from build123d import *

# Parameters (mm, degrees)
SKETCH4_R          = 1
CUT_EXTRUDE1_DEPTH = 2
SKETCH5_R          = 1
CUT_EXTRUDE2_DEPTH = 10


with BuildPart() as part:
    # Sketch1 → Revolve1 (revolve)
    with BuildSketch(Plane.XY, mode=Mode.PRIVATE) as revolve1_sk:
        with BuildLine():
            Line((0, 0.8346352), (25, 0.8346352))
            Line((25, 0.8346352), (25, -1.1653648))
            Line((25, -1.1653648), (-3, -1.1653648))
            ThreePointArc((-3, -1.1653648), (-1.802775638, 0.288798657), (0, 0.8346352))
        make_face()
    revolve(revolve1_sk.sketch.rotate(Axis((-3, -1.1653648, 0), (1, 0, 0)), 180), axis=Axis((-3, -1.1653648, 0), (1, 0, 0)))

    # Sketch4 → Cut-Extrude1 (cut)
    with BuildSketch(Plane(origin=(0, 0.8346352, 0), x_dir=(1, 0, 0), z_dir=(0, 1, 0))):
        with Locations(Location((21, 0, 0), (0, 0, 180))):
            Circle(SKETCH4_R)
    extrude(amount=-CUT_EXTRUDE1_DEPTH, mode=Mode.SUBTRACT)

    # Sketch5 → Cut-Extrude2 (cut)
    with BuildSketch(Plane(origin=(25, 0, 0), x_dir=(0, 0, -1), z_dir=(1, 0, 0))):
        with Locations(Location((0, -1.1653648, 0), (0, 0, 90))):
            Circle(SKETCH5_R)
    extrude(amount=-CUT_EXTRUDE2_DEPTH, mode=Mode.SUBTRACT)


solid = part.part
Source: CAD feature listing. Evaluate the final solid. Frame: model axes, mm. A direction names the side the tool comes from. Give positions to 0.01 mm unless a question says otherwise; leave off trailing zeros. Write each loop counter-clockwise with the first axis right and the second up, starting at its lowest first coordinate (ties: lowest second). Pieces come first, ordered by that corner, then holes. Notation, with made-up numbers: M 52,40.25 L 111,40.25 A19 ccw 111,76.25 Z; hole C -37,7 d4. An arc over 180 degrees is marked long. Return JSON: item names as keys, results as strings. Group by question number.
1) Ray query, L1, parallel to X at y = -0.5, z = 0.8; L2, parallel to Y at x = 19.75, z = 0.7; L3, parallel to Y at x = 23, z = -0.55. Return the intervals inside material, ascending.
2) First-contact query: pin 1 Ø2 at (x, z) = (18.5, 1) entering from -Y; pin 2 Ø1 at (y, z) = (-1, 0) entering from +X; pin 3 Ø1.5 at (x, z) = (16.5, -1) entering from -Y. Flat tips, straight axial feed; report the tip coordinate or a pass-through.
3) Cut plane C-C, the plane x = 21. Output: boundary loops of the cut face in (y, z), then the cut area to 3 significant figures.
4) Set-up query: faces 1 (the face through (20.07, -2.164, 0.044)), 2 (the face through (20, 0, 0)). Return all of +Z, -Z, +X, -X, +Y, -Y with unobstructed straight access to the full face (end or side cutting, diameter ignored); none if empty.
5) Cut plane A-A, the plane x = 15.5. Output: boundary loops of the cut face in (y, z), then the cut area to 3 significant figures.
6) Cut plane B-B, the plane x = 6.25. Output: boundary loops of the cut face in (y, z).
7) Draft query along Z for faces 3 (the face through (12.7, -3, 0.8)), 4 (the face through (15, -1, 0)), 5 (the face through (25, -2, -1)). Return one class per face: released by +Z, released by -Z, zero draft, split by the parting line, or undercut.
Data:
{
 "1": {"L1": "x = -2.31 to 20.4, 21.6 to 25", "L2": "y = -3.04 to -1.88, -0.45 to 0.71", "L3": "y = -3.09 to -2, -0.33 to 0.76"},
 "2": {"pin 1": "stops at y = -3.17", "pin 2": "stops at x = 15", "pin 3": "stops at y = -3.15"},
 "3": {"outline": "M -1.17,-1 A1 cw -1.17,1 L 0.57,1 A2 ccw long 0.57,-1 Z", "area": "7.17 mm²"},
 "4": {"face 1": "+X", "face 2": "+Y"},
 "5": {"outline": "C -1.17,0 d4; hole C -1.17,0 d2", "area": "9.42 mm²"},
 "6": {"outline": "C -1.17,0 d4"},
 "7": {"face 3": "split by the parting line", "face 4": "undercut", "face 5": "zero draft"}
}
